Here's how the part is built. I have some questions about the finished solid (model axes, mm). A direction names the side the tool comes from. Give positions to 0.01 mm unless a question says otherwise; leave off trailing zeros. Loops run counter-clockwise (first coordinate to the right, second up) from the corner with the lowest first, then second, coordinate; pieces in that order, holes last. Notation, with made-up numbers: (9.5, 15.25) - (24.5, 15.25) arc R31 ccw to (24.5, 47.25) - close; hole circle Ø10 at (62, 48). An arc over 180 degrees is marked (long way). Use a Markdown table: item, result.
from build123d import *

# Parameters (mm, degrees)
SKETCH_1_W          = 12
SKETCH_1_H          = 12
EXTRUDE_1_DEPTH     = 50
SKETCH_2_W          = 10
SKETCH_2_H          = 10
CUT_EXTRUDE_1_DEPTH = 47.5
SKETCH_3_R          = 2.1
CUT_EXTRUDE_2_DEPTH = 47.5
SKETCH_5_R          = 3.05
CUT_EXTRUDE_4_DEPTH = 47.5


with BuildPart() as part:
    # ｽｹｯﾁ1 → ﾎﾞｽ - 押し出し1 (new body)
    with BuildSketch(Plane.XY):
        Rectangle(SKETCH_1_W, SKETCH_1_H)
    extrude(amount=EXTRUDE_1_DEPTH)

    # ｽｹｯﾁ2 → ｶｯﾄ - 押し出し1 (cut)
    with BuildSketch(Plane.XY.offset(50)):
        Rectangle(SKETCH_2_W, SKETCH_2_H)
    extrude(amount=-CUT_EXTRUDE_1_DEPTH, mode=Mode.SUBTRACT)

    # ｽｹｯﾁ3 → ｶｯﾄ - 押し出し2 (cut)
    with BuildSketch(Plane(origin=(0, 6, 0), x_dir=(1, 0, 0), z_dir=(0, 1, 0))):
        with Locations((0, -10)):
            Circle(SKETCH_3_R)
        with Locations((0, -40)):
            Circle(SKETCH_3_R)
    extrude(amount=-CUT_EXTRUDE_2_DEPTH, mode=Mode.SUBTRACT)

    # ｽｹｯﾁ5 → ｶｯﾄ - 押し出し4 (cut)
    with BuildSketch(Plane.ZY.offset(6)):
        with Locations((40, 0)):
            Circle(SKETCH_5_R)
    extrude(amount=-CUT_EXTRUDE_4_DEPTH, mode=Mode.SUBTRACT)


solid = part.part
(1) Will these pins go through, and if not, where does the flat tip stop? pin 1 (1.5 mm diameter, centred on x = -1.5, y = 1.5, fed in from +Z); pin 2 (5 mm diameter, centred on x = 0, z = 40, fed in from +Y).
A:
| item | result |
|---|---|
| pin 1 | z = 2.5 |
| pin 2 | y = 6 |
(2) Suppose I cut it at C-C on y = 0. Write out the boundary of the cut face in (x, z).
A:
| item | result |
|---|---|
| outline | (-6, 0) - (6, 0) - (6, 36.95) - (5, 36.95) - (5, 2.5) - (-5, 2.5) - (-5, 36.95) - (-6, 36.95) - close; (-6, 43.05) - (-5, 43.05) - (-5, 50) - (-6, 50) - close; (5, 43.05) - (6, 43.05) - (6, 50) - (5, 50) - close |
(3) If I drill on line 1 (Z direction, x = 0, y = 5.3); line 2 (Y direction, x = 4.5, z = 4.5), over which ranges is the centre line in solid material (lowest first)?
A:
| item | result |
|---|---|
| line 1 | 0 to 7.9, 12.1 to 37.9, 42.1 to 50 |
| line 2 | -6 to -5, 5 to 6 |
(4) Suppose I cut it at A-A on x = 0. Write out the boundary of the cut face in (y, z), plus the area to 3 significant figures.
A:
| item | result |
|---|---|
| outline | (-6, 0) - (6, 0) - (6, 7.9) - (5, 7.9) - (5, 2.5) - (-5, 2.5) - (-5, 7.9) - (-6, 7.9) - close; (-6, 12.1) - (-5, 12.1) - (-5, 37.9) - (-6, 37.9) - close; (-6, 42.1) - (-5, 42.1) - (-5, 50) - (-6, 50) - close; (5, 12.1) - (6, 12.1) - (6, 37.9) - (5, 37.9) - close; (5, 42.1) - (6, 42.1) - (6, 50) - (5, 50) - close |
| area | 108 mm2 |
(5) On a 3-axis mill with a long thin cutter (end or side, diameter ignored), from which of +Z, -Z, +X, -X, +Y, -Y can I reach the whole of each face in a straight line? I mean faces 1 (the face through (0, 0, 2.5)), 2 (the face through (-5.507, -1.168, 42.817)). Say none if no direction works.
A:
| item | result |
|---|---|
| face 1 | +Z |
| face 2 | +X, -X |
(6) Suppose I cut it at D-D on x = 3.75. Write out the boundary of the cut face in (y, z).
A:
| item | result |
|---|---|
| outline | (-6, 0) - (6, 0) - (6, 50) - (5, 50) - (5, 2.5) - (-5, 2.5) - (-5, 50) - (-6, 50) - close |
(7) We'd pull the mould along X, two halves only. Please class faces 3 (the face through (0, 5, 27)), 4 (the face through (-6, 0, 25)), 5 (the face through (5.2, 0.1, 50)), 6 (the face through (6, 0, 25)): pulls with the +X half, pulls with the -X half, needs draft (parallel to the pull), parting line crosses it, or undercut.
A:
| item | result |
|---|---|
| face 3 | undercut |
| face 4 | pulls with the -X half |
| face 5 | needs draft |
| face 6 | pulls with the +X half |
(8) Suppose I cut it at B-B on z = 6. Write out the boundary of the cut face in (x, y).
A:
| item | result |
|---|---|
| outline | (-6, -6) - (6, -6) - (6, 6) - (-6, 6) - close; hole (-5, -5) - (5, -5) - (5, 5) - (-5, 5) - close |
